from build123d import *

# Parameters (mm, degrees)
F1_DEPTH      = 2.5
F3_DEPTH      = 2.7
F4_R          = 1
F5_R          = 5
F6_W          = 4
F6_H          = 2
F6_H_2        = 4
F7_DEPTH      = 2
F8_R          = 1.5
F9_DEPTH      = 6
F10_R         = 2.5
F11_DEPTH     = 3.5
F12_S5_R      = 1.5
F12_T6_DEPTH  = 5
F12_S11_R     = 1.5
F12_T12_DEPTH = 5
F13_SIZE      = 0.5


# Not quite as in the source:
# - a fillet or chamfer that OpenCascade refuses, or shapes differently, is made with other operations: its cross-section is extruded or revolved along the edge and cut away or added


with BuildPart() as f1:
    # F0 (on Top) → F1 (new body)
    with BuildSketch(Plane.XY):
        Polygon((55, 0), (4, 0), (0, -10), (0, -47), (59, -47), (59, -10), align=None)
    extrude(amount=F1_DEPTH)

    # F2 (on face) → F3 (join)
    with BuildSketch(Plane.XY.offset(2.5)):
        with BuildLine():
            Line((0, -39.5), (0, -47))
            Line((0, -47), (59, -47))
            Line((59, -47), (59, -39.5))
            Line((59, -39.5), (53.5, -32))
            Line((53.5, -32), (53.5, -4))
            ThreePointArc((53.5, -4), (52.3284271247, -1.1715728753), (49.5, 0))
            Line((49.5, 0), (9.5, 0))
            ThreePointArc((9.5, 0), (6.6715728753, -1.1715728753), (5.5, -4))
            Line((5.5, -4), (5.5, -32))
            Line((5.5, -32), (0, -39.5))
        make_face()
    extrude(amount=F3_DEPTH)

    # F4
    f4_edges = [f1.edges().sort_by_distance(p)[0] for p in [
        (0, -47, 2.6),
        (59, -47, 2.6),
        (4, 0, 1.25),
        (55, 0, 1.25),
        (59, -10, 1.25),
        (0, -10, 1.25),
    ]]
    fillet(f4_edges, radius=F4_R)

    # F5
    f5_edges = [f1.edges().sort_by_distance(p)[0] for p in [
        (0, -39.5, 3.85),
        (59, -39.5, 3.85),
        (53.5, -32, 3.85),
        (5.5, -32, 3.85),
    ]]
    fillet(f5_edges, radius=F5_R)

    # F6 (on face) → F7 (join)
    with BuildSketch(Plane.XY.offset(5.2)):
        with Locations((11.5, -5)):
            Rectangle(F6_W, F6_H)
        with Locations((11.5, -41)):
            Rectangle(F6_W, F6_H_2)
        with Locations((47.5, -5)):
            Rectangle(F6_W, F6_H)
        with Locations((47.5, -41)):
            Rectangle(F6_W, F6_H_2)
    extrude(amount=F7_DEPTH)

    # F8 (on face) → F9 (cut)
    with BuildSketch(Plane.XY.offset(5.2)):
        with Locations((23.5, -16.5)):
            Circle(F8_R)
        with Locations((35.5, -16.5)):
            Circle(F8_R)
    extrude(amount=-F9_DEPTH, mode=Mode.SUBTRACT)

    # F10 (on face) → F11 (cut)
    with BuildSketch(Plane.XY):
        with Locations((35.5, -16.5)):
            Circle(F10_R)
        with Locations((23.5, -16.5)):
            Circle(F10_R)
    extrude(amount=F11_DEPTH, mode=Mode.SUBTRACT)

    # F12: chamfer of 1.2 on 2 edges, made by hand


with BuildPart() as f12_tool2:
    # F12_s3 → F12_t4 (revolve)
    with BuildSketch(Plane.XZ.offset(16.5)):
        Polygon((38, 2.3), (36.8, 3.5), (38, 3.5), align=None)
    revolve(axis=Axis((35.5, -16.5, 3.5), (0, 0, 1)))

    # F12_s5 → F12_t6 (cut, symmetric)
    with BuildSketch(Plane.XY.offset(2.9)):
        with Locations((35.5, -16.5)):
            Circle(F12_S5_R)
    extrude(amount=F12_T6_DEPTH, both=True, mode=Mode.SUBTRACT)


with BuildPart() as f1_1:
    add(f1.part)

    # F12_t1: union F12_tool2
    add(f12_tool2.part)


with BuildPart() as f12_tool8:
    # F12_s9 → F12_t10 (revolve)
    with BuildSketch(Plane.XZ.offset(16.5)):
        Polygon((26, 2.3), (24.8, 3.5), (26, 3.5), align=None)
    revolve(axis=Axis((23.5, -16.5, 3.5), (0, 0, 1)))

    # F12_s11 → F12_t12 (cut, symmetric)
    with BuildSketch(Plane.XY.offset(2.9)):
        with Locations((23.5, -16.5)):
            Circle(F12_S11_R)
    extrude(amount=F12_T12_DEPTH, both=True, mode=Mode.SUBTRACT)


with BuildPart() as f1_2:
    add(f1_1.part)

    # F12_t7: union F12_tool8
    add(f12_tool8.part)

    # F13
    f13_edges = [f1_2.edges().sort_by_distance(p)[0] for p in [
        (29.5, 0, 0),
        (54.883596, -0.171933, 0),
        (4.116404, -0.171933, 0),
        (57.08996, -5.224901, 0),
        (1.91004, -5.224901, 0),
        (58.981956, -10.003475, 0),
        (0.018044, -10.003475, 0),
        (59, -28.096291, 0),
        (0, -28.096291, 0),
        (58.707107, -46.707107, 0),
        (0.292893, -46.707107, 0),
        (29.5, -47, 0),
        (21, -16.5, 0),
        (33, -16.5, 0),
    ]]
    chamfer(f13_edges, length=F13_SIZE)


solid = f1_2.part
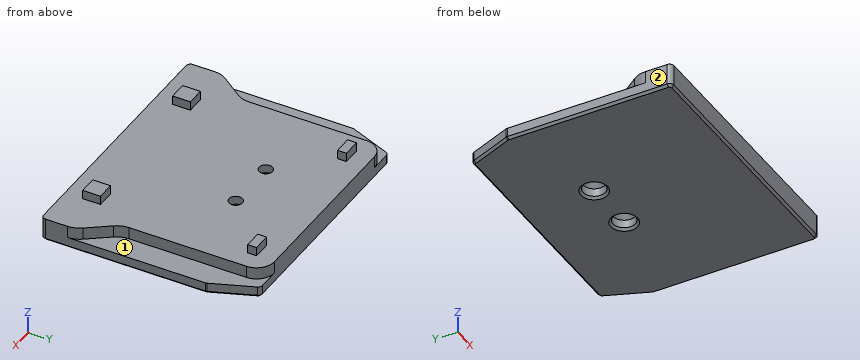
Check sheet for the modelled part. Datum: model origin and axes. Units: mm. Face numbers are marked on the shaded views. A direction names the side the tool comes from. Round coordinates to 2 decimals unless told otherwise and drop trailing zeros. Write each loop counter-clockwise with the first axis right and the second up, starting at its lowest first coordinate (ties: lowest second). Pieces come first, ordered by that corner, then holes. Notation, with made-up numbers: (-19.5, 7.25) -> (23.5, 7.25) arc R13 cw to (23.5, 30.25) -> close; hole circle Ø7 at (18.25, 88.5). An arc over 180 degrees is marked (long way). Answer as CSV lines item,"result". Start each with the question number.
1) Section check D-D on x = 12. Enter the section's corners in (y, z), and give its area (3 significant figures).
2) Section check B-B on x = 35.5. Enter the section's corners in (y, z), and give its area (3 significant figures).
3) Section check C-C on z = 1.5. Enter the section's corners in (x, y), and give its area (3 significant figures).
4) Material ranges on line 1 (Y direction, x = 35.5, z = 3.85); line 2 (Y direction, x = 49, z = 5.5); line 3 (Z direction, x = 52, y = -24), recorded low to high. Write a range as from..to.
5) Go/stop test with flat-tipped pins: P1, Ø10.5, axis at x = 52.5, y = -27, coming from the +Z side; P2, Ø1, axis at y = -36, z = 4.5, coming from the +X side; P3, Ø0.8, axis at y = -18, z = 4.5, coming from the -X side. Record where each tip stops, or that it passes through.
6) Section check A-A on y = -16.5. State how many separate pieces and enclosed holes the cut face has, and give its area (3 significant figures).
7) Tool access check on the marked faces 1 and 2. Record the directions out of +Z, -Z, +X, -X, +Y, -Y that give a thin tool (end or side, any length) a straight path to the whole face; none if there is none.
Found:
1,outline,"(-47, 0.5) -> (-46.5, 0) -> (-0.5, 0) -> (0, 0.5) -> (0, 5.2) -> (-4, 5.2) -> (-4, 7.2) -> (-6, 7.2) -> (-6, 5.2) -> (-39, 5.2) -> (-39, 7.2) -> (-43, 7.2) -> (-43, 5.2) -> (-47, 5.2) -> close"
1,area,"256 mm^2"
2,outline,"(-47, 0.5) -> (-46.5, 0) -> (-19.5, 0) -> (-19, 0.5) -> (-19, 2.3) -> (-18, 3.3) -> (-18, 5.2) -> (-47, 5.2) -> close; (-15, 3.3) -> (-14, 2.3) -> (-14, 0.5) -> (-13.5, 0) -> (-0.5, 0) -> (0, 0.5) -> (0, 5.2) -> (-15, 5.2) -> close"
2,area,"223 mm^2"
3,outline,"(0, -46) arc R1 ccw to (1, -47) -> (58, -47) arc R1 ccw to (59, -46) -> (59, -10.19) arc R1 ccw to (58.93, -9.82) -> (55.25, -0.63) arc R1 ccw to (54.32, 0) -> (4.68, 0) arc R1 ccw to (3.75, -0.63) -> (0.07, -9.82) arc R1 ccw to (0, -10.19) -> close; hole circle Ø5 at (23.5, -16.5); hole circle Ø5 at (35.5, -16.5)"
3,area,"2,690 mm^2"
4,line 1,"y = -47..-18, -15..0"
4,line 2,"y = -43..-39, -6..-4"
4,line 3,"z = 0..5.2"
5,P1,"stops at z = 5.2"
5,P2,"stops at x = 56.8"
5,P3,"stops at x = 5.5"
6,separate pieces,"3"
6,enclosed holes,"0"
6,area,"234 mm^2"
7,face 1,"+Z, +X, +Y"
7,face 2,"+Z, -Z, -X, +Y, -Y"
